```python
from build123d import *

# Parameters (mm, degrees)
F2_W     = 50.8
F2_H     = 50.8
F0_W     = 101.6
F0_H     = 101.6
F4_R     = 19.05
F5_DEPTH = 12.7


with BuildPart() as f3:
    # F2 (on offset) → F3 section 0
    with BuildSketch(Plane.XY.offset(76.2)):
        Rectangle(F2_W, F2_H)
    # F0 (on Top) → F3 section 1
    with BuildSketch(Plane.XY):
        Rectangle(F0_W, F0_H)
    loft()

    # F4 (on face) → F5 (cut)
    with BuildSketch(Plane.XY.offset(76.2)):
        Circle(F4_R)
    extrude(amount=-F5_DEPTH, mode=Mode.SUBTRACT)


solid = f3.part
```
For this review, take the finished solid that the model builds, in its own axes (mm). Round coordinates to 2 decimals unless told otherwise and drop trailing zeros. Use CSV: the item, a comma, the result in double quotes.
1) Wall thickness on line 1 along X through (y, z) = (-1.5, 69); line 2 along Y through (x, z) = (-6, 71); line 3 along Y through (x, z) = (0, 68.25): over which ranges is each line inside the solid? List them lowest first. Write a range as from..to.
Conclusion:
line 1,"x = -27.8..-18.99, 18.99..27.8"
line 2,"y = -27.13..-18.08, 18.08..27.13"
line 3,"y = -28.05..-19.05, 19.05..28.05"
2) The part is to be moulded in two halves that separate along X. For faces 1 (the flat face through (0, 0, 63.5)), 2 (the flat face through (-1, 0, 0)), 3 (the cylindrical face through (-15.12, -11.59, 69.94)), say which applies: pulls with the +X half, pulls with the -X half, needs draft (parallel to the pull), parting line crosses it, or undercut.
Conclusion:
face 1,"undercut"
face 2,"needs draft"
face 3,"undercut"
3) Clearance check with flat-ended pins moving along their axes: pin 1 Ø5 at (y, z) = (-18, 39.5) entering from +X; pin 2 Ø12 at (x, z) = (11.5, 49) entering from +Y; pin 3 Ø12 at (x, y) = (-9, 25.5) entering from -Z; pin 4 Ø3 at (y, z) = (28.5, 61) entering from -X. State where each tip first meets the part, or that it passes through.
Conclusion:
pin 1,"stops at x = 38.47"
pin 2,"stops at y = 36.47"
pin 3,"stops at z = 0"
pin 4,"stops at x = -30.97"
